Input: part model. Units: mm. Frame: model coordinates. Round coordinates to 2 decimals unless told otherwise and drop trailing zeros. Write each loop counter-clockwise with the first axis right and the second up, starting at its lowest first coordinate (ties: lowest second). Pieces come first, ordered by that corner, then holes. Notation, with made-up numbers: (-7.5, 17) -> (4.5, 17) arc R9 cw to (4.5, 29) -> close; hole circle Ø11 at (41, 75). An arc over 180 degrees is marked (long way). Write item = value, one per line.
```python
from build123d import *

# Parameters (mm, degrees)
EXTRUDE_1_DEPTH = 4
CHAMFER_1_SIZE  = 10
CHAMFER_2_SIZE  = 2
CHAMFER_3_SIZE  = 2


with BuildPart() as part:
    # Эскиз1 → Бобышка-Вытянуть1 (new, symmetric)
    with BuildSketch(Plane.XY):
        Polygon((0, 0), (0, 52), (8, 52), (70, 8), (70, 0), align=None)
    extrude(amount=EXTRUDE_1_DEPTH, both=True)

    # Фаска1
    chamfer_1_edges = [part.edges().sort_by_distance(p)[0] for p in [
        (0, 0, 0),
    ]]
    chamfer(chamfer_1_edges, length=CHAMFER_1_SIZE)

    # Фаска2
    chamfer_2_edges = [part.edges().sort_by_distance(p)[0] for p in [
        (0, 31, 4),
        (0, 31, -4),
    ]]
    chamfer(chamfer_2_edges, length=CHAMFER_2_SIZE)

    # Фаска3
    chamfer_3_edges = [part.edges().sort_by_distance(p)[0] for p in [
        (0, 52, 0),
    ]]
    chamfer(chamfer_3_edges, length=CHAMFER_3_SIZE)


solid = part.part
```
1) Cut plane D-D (x = 7). Return the cut outline in (y, z).
Solutions:
outline = (3, -4) -> (52, -4) -> (52, 4) -> (3, 4) -> close
2) Line query: L1, parallel to Y at x = 6, z = -2.75; L2, parallel to X at y = 2, z = -1; L3, parallel to Y at x = 21.5, z = -3. Output: solid intervals per line, ascending. Write a range as from..to.
Solutions:
L1 = 4..52
L2 = 8..70
L3 = 0..42.42
3) Cut plane A-A (z = -3). Return the cut outline in (x, y).
Solutions:
outline = (1, 9) -> (10, 0) -> (70, 0) -> (70, 8) -> (8, 52) -> (2, 52) -> (1, 51) -> close
4) Cut plane C-C (z = 0.75). Return the cut outline in (x, y).
Solutions:
outline = (0, 10) -> (10, 0) -> (70, 0) -> (70, 8) -> (8, 52) -> (2, 52) -> (0, 50) -> close
5) First-contact query: P1, Ø2, axis at y = 38.5, z = -0.5, coming from the +X side; P2, Ø2, axis at y = 20, z = -2.5, coming from the +X side. Flat tips, straight axial feed; report the tip coordinate or a pass-through.
Solutions:
P1 = 28.43
P2 = 54.5
6) Cut plane B-B (y = 4.5). Return the cut outline in (x, z), and give its area (3 significant figures).
Solutions:
outline = (5.5, -4) -> (70, -4) -> (70, 4) -> (5.5, 4) -> close
area = 516 mm^2
